Geometry: final body of the model. Coordinates: model frame, mm. Face numbers are marked on the shaded views. Give positions to 0.01 mm unless a question says otherwise; leave off trailing zeros. Write each loop counter-clockwise with the first axis right and the second up, starting at its lowest first coordinate (ties: lowest second). Pieces come first, ordered by that corner, then holes.
Q1. Draft query along X for the marked faces 1, 2 and 3. Return one class per face: pulls with the +X half, pulls with the -X half, needs draft (parallel to the pull), parting line crosses it, or undercut.
Q2. Pin query (flat end, axial travel): pin 1 (1.7 mm diameter, centred on x = 0.5, z = 9, fed in from -Y); pin 2 (3 mm diameter, centred on x = -6, z = 11, fed in from -Y). Return the tip coordinate at first contact, or that it passes through.
Q3. Cut plane A-A on x = 0. Return the cut outline in (y, z), plus the area to 3 significant figures.
Q4. Line query: L1, parallel to X at y = 0, z = 5.5; L2, parallel to X at y = 4.5, z = 1; L3, parallel to Y at x = 0, z = 5.5. Output: solid intervals per line, ascending.
Q5. Cut plane C-C on y = -4.5. Return the cut outline in (x, z), plus the area to 3 significant figures.
Q6. Cut plane B-B on y = 6.75. Return the cut outline in (x, z), plus the area to 3 significant figures.
```python
from build123d import *

# Parameters (mm, degrees)
BOSS_EXTRUDE1_DEPTH = 12.7
CUT_EXTRUDE1_REACH  = 19.791


with BuildPart() as part:
    # Sketch1 → Boss-Extrude1 (new body)
    with BuildSketch(Plane.XY):
        with BuildLine():
            ThreePointArc((-7.16977096, 5.440072093), (-7.281152949, 5.290067271), (-7.389397086, 5.137782665))
            ThreePointArc((-7.389397086, 5.137782665), (-6.616232826, 3.46280058), (-5.009138832, 2.556932568))
            ThreePointArc((-5.009138832, 2.556932568), (-5.348741848, 1.737911576), (-5.555405697, 0.875696031))
            ThreePointArc((-5.555405697, 0.875696031), (-7.388027907, 1.087459563), (-8.9980607, 0.186825141))
            ThreePointArc((-8.9980607, 0.186825141), (-9, 0), (-8.9980607, -0.186825141))
            ThreePointArc((-8.9980607, -0.186825141), (-7.388027907, -1.087459563), (-5.555405697, -0.875696031))
            ThreePointArc((-5.555405697, -0.875696031), (-5.348741848, -1.737911576), (-5.009138832, -2.556932568))
            ThreePointArc((-5.009138832, -2.556932568), (-6.616232826, -3.46280058), (-7.389397086, -5.137782665))
            ThreePointArc((-7.389397086, -5.137782665), (-7.281152949, -5.290067271), (-7.16977096, -5.440072093))
            ThreePointArc((-7.16977096, -5.440072093), (-5.337847438, -5.222347115), (-3.979696407, -3.97383851))
            ThreePointArc((-3.979696407, -3.97383851), (-3.305704259, -4.549911576), (-2.549551188, -5.012899834))
            ThreePointArc((-2.549551188, -5.012899834), (-3.317261682, -6.690388598), (-2.958234941, -8.49993212))
            ThreePointArc((-2.958234941, -8.49993212), (-2.781152949, -8.559508647), (-2.602872405, -8.615396407))
            ThreePointArc((-2.602872405, -8.615396407), (-1.248790674, -7.362475569), (-0.883878355, -5.554109745))
            ThreePointArc((-0.883878355, -5.554109745), (0, -5.624), (0.883878355, -5.554109745))
            ThreePointArc((0.883878355, -5.554109745), (1.248790674, -7.362475569), (2.602872405, -8.615396407))
            ThreePointArc((2.602872405, -8.615396407), (2.781152949, -8.559508647), (2.958234941, -8.49993212))
            ThreePointArc((2.958234941, -8.49993212), (3.317261682, -6.690388598), (2.549551188, -5.012899834))
            ThreePointArc((2.549551188, -5.012899834), (3.305704259, -4.549911576), (3.979696407, -3.97383851))
            ThreePointArc((3.979696407, -3.97383851), (5.337847438, -5.222347115), (7.16977096, -5.440072093))
            ThreePointArc((7.16977096, -5.440072093), (7.281152949, -5.290067271), (7.389397086, -5.137782665))
            ThreePointArc((7.389397086, -5.137782665), (6.616232826, -3.46280058), (5.009138832, -2.556932568))
            ThreePointArc((5.009138832, -2.556932568), (5.348741848, -1.737911576), (5.555405697, -0.875696031))
            ThreePointArc((5.555405697, -0.875696031), (7.388027907, -1.087459563), (8.9980607, -0.186825141))
            ThreePointArc((8.9980607, -0.186825141), (9, 0), (8.9980607, 0.186825141))
            ThreePointArc((8.9980607, 0.186825141), (7.388027907, 1.087459563), (5.555405697, 0.875696031))
            ThreePointArc((5.555405697, 0.875696031), (5.348741848, 1.737911576), (5.009138832, 2.556932568))
            ThreePointArc((5.009138832, 2.556932568), (6.616232826, 3.46280058), (7.389397086, 5.137782665))
            ThreePointArc((7.389397086, 5.137782665), (7.281152949, 5.290067271), (7.16977096, 5.440072093))
            ThreePointArc((7.16977096, 5.440072093), (5.337847438, 5.222347115), (3.979696407, 3.97383851))
            ThreePointArc((3.979696407, 3.97383851), (3.305704259, 4.549911576), (2.549551188, 5.012899834))
            ThreePointArc((2.549551188, 5.012899834), (3.317261682, 6.690388598), (2.958234941, 8.49993212))
            ThreePointArc((2.958234941, 8.49993212), (2.781152949, 8.559508647), (2.602872405, 8.615396407))
            ThreePointArc((2.602872405, 8.615396407), (1.248790674, 7.362475569), (0.883878355, 5.554109745))
            ThreePointArc((0.883878355, 5.554109745), (0, 5.624), (-0.883878355, 5.554109745))
            ThreePointArc((-0.883878355, 5.554109745), (-1.248790674, 7.362475569), (-2.602872405, 8.615396407))
            ThreePointArc((-2.602872405, 8.615396407), (-2.781152949, 8.559508647), (-2.958234941, 8.49993212))
            ThreePointArc((-2.958234941, 8.49993212), (-3.317261682, 6.690388598), (-2.549551188, 5.012899834))
            ThreePointArc((-2.549551188, 5.012899834), (-3.305704259, 4.549911576), (-3.979696407, 3.97383851))
            ThreePointArc((-3.979696407, 3.97383851), (-5.337847438, 5.222347115), (-7.16977096, 5.440072093))
        make_face()
    extrude(amount=BOSS_EXTRUDE1_DEPTH)

    # Sketch2 → Cut-Extrude1 (cut, up to next)
    with BuildSketch(Plane.XY.offset(12.7), mode=Mode.PRIVATE) as cut_extrude1_sk1:
        with BuildLine():
            Line((1.669458355, 1.6891), (-1.669458355, 1.6891))
            ThreePointArc((-1.669458355, 1.6891), (0, -2.3749), (1.669458355, 1.6891))
        make_face()
    cut_extrude1_tool1 = extrude(cut_extrude1_sk1.sketch, amount=-CUT_EXTRUDE1_REACH, mode=Mode.PRIVATE) & part.part
    add(cut_extrude1_tool1.solids().sort_by_distance((0, -0.192165, 12.7))[0], mode=Mode.SUBTRACT)


solid = part.part
```
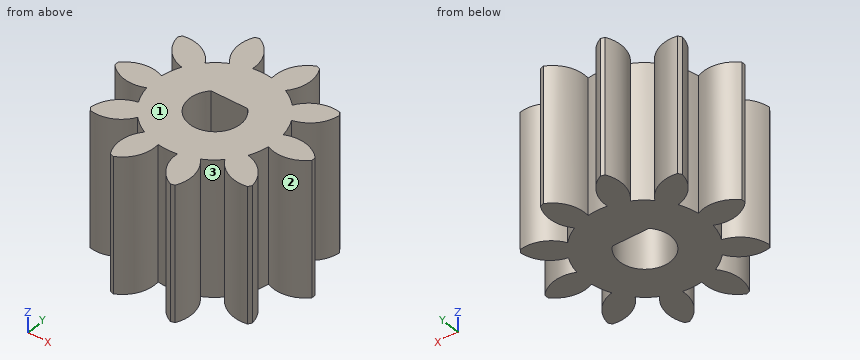
Data:
1. face 1: needs draft
1. face 2: undercut
1. face 3: undercut
2. pin 1: stops at y = -7.53
2. pin 2: stops at y = -5.5
3. outline: (-5.62, 0) - (-2.37, 0) - (-2.37, 12.7) - (-5.62, 12.7) - close; (1.69, 0) - (5.62, 0) - (5.62, 12.7) - (1.69, 12.7) - close
3. area: 91.2 mm2
4. L1: x = -9 to -2.37, 2.37 to 9
4. L2: x = -7.24 to -4.36, -3.37 to 3.37, 4.36 to 7.24
4. L3: y = -5.62 to -2.37, 1.69 to 5.62
5. outline: (-7.24, 0) - (-4.36, 0) - (-4.36, 12.7) - (-7.24, 12.7) - close; (-3.37, 0) - (3.37, 0) - (3.37, 12.7) - (-3.37, 12.7) - close; (4.36, 0) - (7.24, 0) - (7.24, 12.7) - (4.36, 12.7) - close
5. area: 159 mm2
6. outline: (-3.32, 0) - (-0.99, 0) - (-0.99, 12.7) - (-3.32, 12.7) - close; (0.99, 0) - (3.32, 0) - (3.32, 12.7) - (0.99, 12.7) - close
6. area: 59.3 mm2
